```python
from build123d import *

# Parameters (mm, degrees)
F1_DEPTH = 16
F2_W     = 70
F2_H     = 3
F3_DEPTH = 2
F4_W     = 50
F4_H     = 14
F5_DEPTH = 2
F6_R     = 1


with BuildPart() as f1:
    # F0 (on Front) → F1 (new body)
    with BuildSketch(Plane.XZ):
        with BuildLine():
            Line((94, 11), (0, 11))
            ThreePointArc((0, 11), (-11, 0), (0, -11))
            Line((0, -11), (19, -11))
            ThreePointArc((19, -11), (21.7681124643, -11.8361612201), (23.6103896104, -14.064978646))
            ThreePointArc((23.6103896104, -14.064978646), (52.4237101957, -47.6174640031), (95.4149528414, -57.9967593826))
            ThreePointArc((95.4149528414, -57.9967593826), (101.3804745105, -59.0597282402), (106.3380534538, -62.5439444501))
            Line((106.3380534538, -62.5439444501), (107.6335766724, -61))
            ThreePointArc((107.6335766724, -61), (102.0097459375, -57.1560789275), (95.2965735981, -56))
            ThreePointArc((95.2965735981, -56), (53.4811996085, -45.9198240056), (25.4545454545, -13.2909701044))
            ThreePointArc((25.4545454545, -13.2909701044), (22.87535745, -10.1706257081), (19, -9))
            Line((19, -9), (0, -9))
            ThreePointArc((0, -9), (-9, 0), (0, 9))
            Line((0, 9), (94, 9))
            Line((94, 9), (94, 11))
        make_face()
    extrude(amount=F1_DEPTH)

    # F2 (on face) → F3 (join)
    with BuildSketch(Plane.XY.offset(11)):
        with Locations((59, -17.5)):
            Rectangle(F2_W, F2_H)
    extrude(amount=-F3_DEPTH)

    # F4 (on face) → F5 (join)
    with BuildSketch(Plane.XZ.offset(19)):
        with Locations((69, 4)):
            Rectangle(F4_W, F4_H)
    extrude(amount=F5_DEPTH)

    # F6
    f6_edges = [f1.edges().sort_by_distance(p)[0] for p in [
        (69, -21, 11),
        (69, -19, 9),
    ]]
    fillet(f6_edges, radius=F6_R)

    # F7: F1 across plane


with BuildPart() as f1_1:
    add(f1.part)
    add(f1.part.mirror(Plane.XZ))


solid = f1_1.part
```
For this review, take the finished solid that the model builds, in its own axes (mm). A direction names the side the tool comes from. Round coordinates to 2 decimals unless told otherwise and drop trailing zeros. Write each loop counter-clockwise with the first axis right and the second up, starting at its lowest first coordinate (ties: lowest second). Pieces come first, ordered by that corner, then holes. Notation, with made-up numbers: M 7,18 L 63,18 A19 cw 63,35 Z; hole C -3.75,38 d3. An arc over 180 degrees is marked long. One line per item, written item: value. Start each with the question number.
(1) The part is to be moulded in two halves that separate along Z. For faces 1 (the cylindrical face through (22.92, -0.22, -10.2)), 2 (the flat face through (94, 1.5, 9.2)), 3 (the cylindrical face through (102.099, -0.224, -57.192)), 4 (the flat face through (9, 0, -11)), say which applies: released by +Z, released by -Z, zero draft, split by the parting line, or undercut.
(2) We need section D-D (x = 42.5). Give the boundary of the cut face in (y, z), and give its area (3 significant figures).
(3) Insertion check: pin 1 (7 mm diameter, centred on y = 4, z = 2, fed in from +X); pin 2 (1.5 mm diameter, centred on y = 19.5, z = 1.5, fed in from -X); pin 3 (1.6 mm diameter, centred on x = 74, y = -20.5, fed in from -Z). Each pin has a flat end and moves straight along its axis. Give the tip position at first contact, or say it passes through.
(4) We need section A-A (z = 0). Give the boundary of the cut face in (x, y), and give its area (3 significant figures).
(5) Wall thickness on line 1 (Z direction, x = 3, y = -15); line 2 (Z direction, x = 84.5, y = 10); line 3 (Y direction, x = 45, z = 0): over which ranges is each line inside the solid? List them lowest first.
(6) We need section B-B (x = 29.5). Give the boundary of the cut face in (y, z).
(7) We need section C-C (y = 12). Give the boundary of the cut face in (x, z).
(8) Machinability: for faces 5 (the flat face through (26, 16, -17)), 6 (the flat face through (69, -21, 4)), 7 (the flat face through (26, -16, -17)), 8 (the flat face through (10, 0, -9)), 9 (the flat face through (69, 19, 3)), which of the approach directions +Z, -Z, +X, -X, +Y, -Y give a long, thin tool a straight path to every point of the face, cutting with its end or side? Answer none if there is none.
Result:
1. face 1: undercut
1. face 2: zero draft
1. face 3: released by +Z
1. face 4: released by -Z
2. outline: M -19,9 L 19,9 L 19,11 L -19,11 Z; M -16,-40.31 L 16,-40.31 L 16,-37.62 L -16,-37.62 Z
2. area: 162 mm²
3. pin 1: x = -7.12
3. pin 2: x = 44
3. pin 3: z = -3
4. outline: M -11,-16 L -9,-16 L -9,16 L -11,16 Z; M 44,-21 L 94,-21 L 94,-19 L 44,-19 Z; M 44,19 L 94,19 L 94,21 L 44,21 Z
4. area: 264 mm²
5. line 1: -11 to -9, 9 to 11
5. line 2: -57.99 to -55.98, 9 to 11
5. line 3: -21 to -19, 19 to 21
6. outline: M -19,9 L 19,9 L 19,11 L -19,11 Z; M -16,-25.24 L 16,-25.24 L 16,-21.41 L -16,-21.41 Z
7. outline: M 0,-11 L 19,-11 A5 cw 23.61,-14.06 A72 ccw 95.41,-58 A14 cw 106.34,-62.54 L 107.63,-61 A16 ccw 95.3,-56 A70 cw 25.45,-13.29 A7 ccw 19,-9 L 0,-9 A9 cw 0,9 L 94,9 L 94,11 L 0,11 A11 ccw Z
8. face 5: -Z, -X, +Y
8. face 6: +Z, -Z, +X, -X, -Y
8. face 7: -Z, -X, -Y
8. face 8: +X, +Y, -Y
8. face 9: -Z, +X, -X
